```python
from build123d import *

# Parameters (mm, degrees)
F0_R     = 45
F0_R_2   = 10
F1_DEPTH = 10
F2_R     = 36.5
F3_DEPTH = 9
F4_SIZE2 = 2
F4_SIZE  = 25
F5_R     = 2


with BuildPart() as f1:
    # F0 (on Top) → F1 (new body)
    with BuildSketch(Plane.XY):
        Circle(F0_R)
        Circle(F0_R_2, mode=Mode.SUBTRACT)
    extrude(amount=F1_DEPTH)

    # F2 (on face) → F3 (cut)
    with BuildSketch(Plane.XY.offset(10)):
        Circle(F2_R)
    extrude(amount=-F3_DEPTH, mode=Mode.SUBTRACT)

    # F4
    f4_edges = [f1.edges().sort_by_distance(p)[0] for p in [
        (-36.5, 0, 1),
    ]]
    f4_side = f1.faces().sort_by_distance((-35.467624, 0, 1))[0]
    chamfer(f4_edges, length=F4_SIZE, length2=F4_SIZE2, reference=f4_side)

    # F5
    f5_edges = [f1.edges().sort_by_distance(p)[0] for p in [
        (-45, 0, 10),
    ]]
    fillet(f5_edges, radius=F5_R)


solid = f1.part
```
Verification items for the finished model (mm, model axes). A direction names the side the tool comes from. Coordinates: 2 decimals unless noted, no trailing zeros. Loops run counter-clockwise (first coordinate to the right, second up) from the corner with the lowest first, then second, coordinate; pieces in that order, holes last. Notation, with made-up numbers: (-2.5, -17.75) - (2.5, -17.75) arc R19 cw to (2.5, 3.25) - close; hole circle Ø6 at (78.25, 1.5). An arc over 180 degrees is marked (long way). Return JSON: item names as keys, results as strings.
1. Go/stop test with flat-tipped pins: pin 1 (2 mm diameter, centred on x = 27.5, z = 8, fed in from +Y); pin 2 (6 mm diameter, centred on x = 32, y = 31, fed in from -Z); pin 3 (18 mm diameter, centred on x = 0, y = 0, fed in from -Z); pin 4 (1.5 mm diameter, centred on x = 27, z = 2.5, fed in from +Y). Record where each tip stops, or that it passes through.
Established:
{"pin 1": "stops at y = 36.37", "pin 2": "stops at z = 0", "pin 3": "passes through", "pin 4": "stops at y = 36.55"}
2. Section check A-A, the plane x = 0. Record the boundary of the cut face in (y, z), then the cut area to 3 significant figures.
Established:
{"outline": "(-45, 0) - (-10, 0) - (-10, 1) - (-11.5, 1) - (-36.5, 3) - (-36.5, 10) - (-43, 10) arc R2 ccw to (-45, 8) - close; (10, 0) - (45, 0) - (45, 8) arc R2 ccw to (43, 10) - (36.5, 10) - (36.5, 3) - (11.5, 1) - (10, 1) - close", "area": "271 mm2"}
3. Thickness scan on L1, parallel to Y at x = 0, z = 7; L2, parallel to Y at x = 14.5, z = 6; L3, parallel to X at y = 23, z = 4.75. Record the ranges inside material, lowest first.
Established:
{"L1": "y = -45 to -36.5, 36.5 to 45", "L2": "y = -42.6 to -33.5, 33.5 to 42.6", "L3": "x = -38.68 to -28.34, 28.34 to 38.68"}
4. Mould release check, pull along X, two halves, no side actions. Record for faces 1 (the cylindrical face through (-2.17, -9.76, 0.49)), 2 (the flat face through (-1, 11, 0)), 3 (the flat face through (-9, 5, 1)), 4 (the cylindrical face through (20.765, -39.923, 3.944)): +X half, -X half, draft (parallel to the pull), parting line (faces both ways), or undercut.
Established:
{"face 1": "undercut", "face 2": "draft", "face 3": "undercut", "face 4": "parting line"}
5. Tool access check on faces 5 (the flat face through (-19, -32, 10)), 6 (the cylindrical face through (-7.912, -35.632, 6.549)). Record the directions out of +Z, -Z, +X, -X, +Y, -Y that give a thin tool (end or side, any length) a straight path to the whole face; none if there is none.
Established:
{"face 5": "+Z, +X, -X, +Y, -Y", "face 6": "+Z"}
6. Section check C-C, the plane z = 5.25. Record the boundary of the cut face in (x, y), then the cut area to 3 significant figures.
Established:
{"outline": "circle Ø90 at (0, 0); hole circle Ø73 at (0, 0)", "area": "2,180 mm2"}
